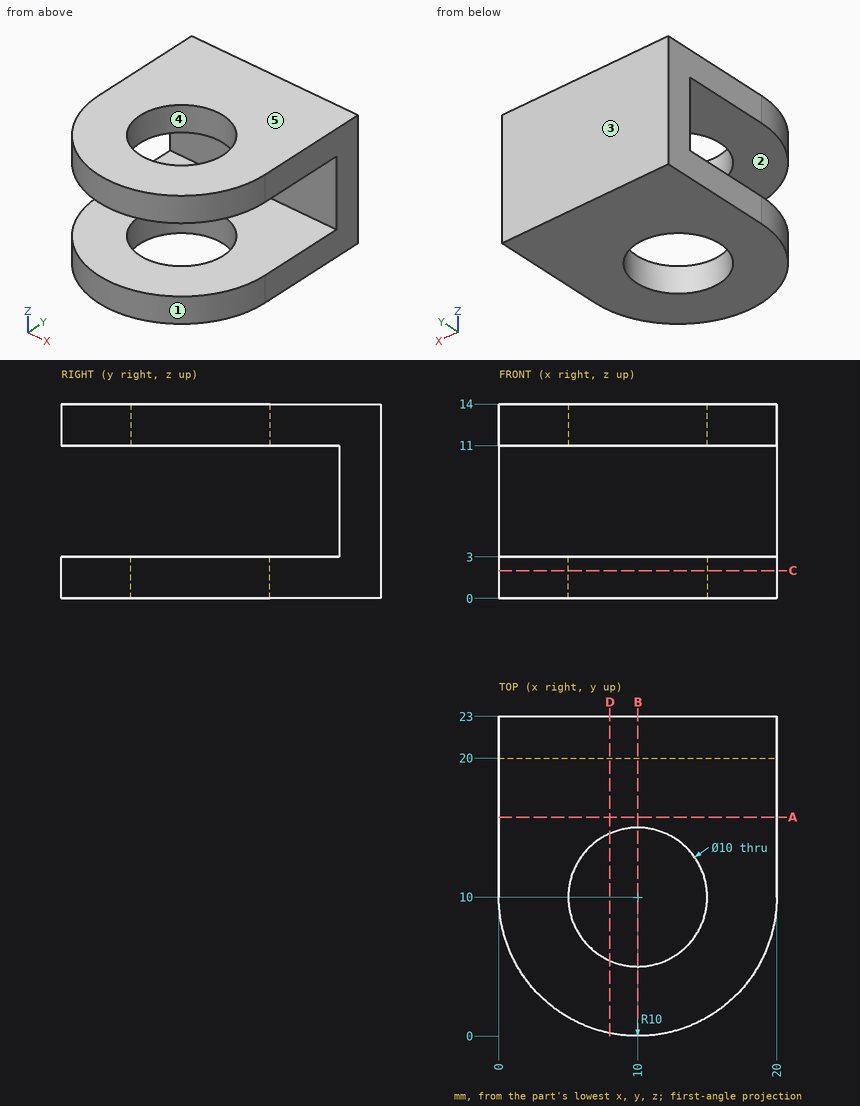
Verification items for this drawing (mm, ordinates from the low corner). A direction names the side the tool comes from. Give positions to 0.01 mm unless a question says otherwise; leave off trailing zeros. Write each loop counter-clockwise with the first axis right and the second up, starting at its lowest first coordinate (ties: lowest second). Pieces come first, ordered by that corner, then holes.
1) Release check for a two-part mould opening along Y. For the marked faces 3, 4 and 5 record: pulls with the +Y half, pulls with the -Y half, needs draft (parallel to the pull), parting line crosses it, or undercut.
2) Section check C-C, the plane z = 2. Record the boundary of the cut face in (x, y).
3) Access from +Z, -Z, +X, -X, +Y, -Y to the whole of each face (thin tool, end or side, straight path). Record for the marked faces 1 and 2.
4) Section check A-A, the plane y = 15.75. Record the boundary of the cut face in (x, z), and give its area (3 significant figures).
5) Section check B-B, the plane x = 10. Record the boundary of the cut face in (y, z).
6) Gauge pin test, flat ends, axial feed: pin 1 (6 mm diameter, centred on x = 11, y = 6.5, fed in from +Z); pin 2 (2 mm diameter, centred on y = 6.5, z = 11, fed in from +X); pin 3 (2.5 mm diameter, centred on x = 8, z = 7.5, fed in from -Y); pin 4 (4 mm diameter, centred on x = 2, z = 9.5, fed in from -Y). Record the tip position at first contact, or that the pin passes through.
7) Material ranges on L1, parallel to Z at x = 2.25, y = 10; L2, parallel to Y at x = 10, z = 13.4; L3, parallel to Y at x = 2.5, z = 5.5, recorded low to high.
8) Section check D-D, the plane x = 8. Record the boundary of the cut face in (y, z), and give its area (3 significant figures).
Computed:
1. face 3: pulls with the +Y half
1. face 4: undercut
1. face 5: needs draft
2. outline: (0, 10) arc R10 ccw to (20, 10) - (20, 23) - (0, 23) - close; hole circle Ø10 at (10, 10)
3. face 1: +Z, -Z, -Y
3. face 2: +X, -X, -Y
4. outline: (0, 0) - (20, 0) - (20, 3) - (0, 3) - close; (0, 11) - (20, 11) - (20, 14) - (0, 14) - close
4. area: 120 mm2
5. outline: (0, 0) - (5, 0) - (5, 3) - (0, 3) - close; (0, 11) - (5, 11) - (5, 14) - (0, 14) - close; (15, 0) - (23, 0) - (23, 14) - (15, 14) - (15, 11) - (20, 11) - (20, 3) - (15, 3) - close
6. pin 1: stops at z = 14
6. pin 2: stops at x = 19.68
6. pin 3: stops at y = 20
6. pin 4: stops at y = 2.56
7. L1: z = 0 to 3, 11 to 14
7. L2: y = 0 to 5, 15 to 23
7. L3: y = 20 to 23
8. outline: (0.2, 0) - (5.42, 0) - (5.42, 3) - (0.2, 3) - close; (0.2, 11) - (5.42, 11) - (5.42, 14) - (0.2, 14) - close; (14.58, 0) - (23, 0) - (23, 14) - (14.58, 14) - (14.58, 11) - (20, 11) - (20, 3) - (14.58, 3) - close
8. area: 106 mm2
